The listing builds one solid part. Answer for the finished solid, in the listing's coordinates (mm). A direction names the side the tool comes from. Give positions to 0.01 mm unless a question says otherwise; leave off trailing zeros. Write each loop counter-clockwise with the first axis right and the second up, starting at its lowest first coordinate (ties: lowest second). Pieces come first, ordered by that corner, then holes. Notation, with made-up numbers: (27, 49) -> (69, 49) arc R17 cw to (69, 56) -> close; hole circle Ø6 at (3, 24.25). An arc over 180 degrees is marked (long way). Put each result on its own line as item: value. Start each with the question number.
1) Find the intervals of material crossed by line 1 along X through (y, z) = (2, -3.5); line 2 along X through (y, z) = (2.3, 14); line 3 along X through (y, z) = (2.6, 5), in increasing order. Write a range as from..to.
2) A cutting plane is placed at C-C (y = 0.8). Give the number of separate pieces and of enclosed holes in the cut face, then the cut area to 3 significant figures.
3) A cutting plane is placed at B-B (x = 7). Write down the section's boundary in (y, z) (3 decimals), then the cut area to 3 significant figures.
4) For a pull along Z with two mould halves and no side action, classify faces 1 (the flat face through (29.366, 1.565, 6.476)), 2 (the flat face through (20.58, 1.57, -4.71)), 3 (the flat face through (28.63, 1.57, 8.7)) as released by +Z, released by -Z, zero draft, split by the parting line, or undercut.
5) A cutting plane is placed at D-D (z = 7.75). Write down the section's boundary in (x, y) (3 decimals), then the cut area to 3 significant figures.
6) Flat-ended cylindrical pins translate along their axes: pin 1 Ø2 at (x, z) = (5.5, 3) entering from -Y; pin 2 Ø1.6 at (x, y) = (-3.5, 1) entering from -Z. Find the tip coordinate at first contact, or state that the pin passes through.
7) A cutting plane is placed at A-A (x = 0.72). Write down the section's boundary in (y, z) (1 decimal).
8) For faces 4 (the cylindrical face through (26.784, 1.565, 8.433)), 5 (the flat face through (24.23, 1.57, -3.77)), 6 (the flat face through (15.044, 1.565, 12.893)), 7 (the flat face through (29.262, 1.565, 2.712)), determine the directions among +Z, -Z, +X, -X, +Y, -Y from which every point of the face is accessible in a straight line to the end or side of a thin tool.
from build123d import *

# Parameters (mm, degrees)
CROQUIS1_R              = 1.5875
SALIENTE_EXTRUIR1_DEPTH = 3.175
SALIENTE_EXTRUIR2_START = -3.175
CROQUIS2_R              = 7.5
CROQUIS2_R_2            = 1.5875
SALIENTE_EXTRUIR2_DEPTH = 3.175
SALIENTE_EXTRUIR3_START = -3.175
SALIENTE_EXTRUIR3_DEPTH = 3.175
CORTAR_EXTRUIR4_START   = -10
CORTAR_EXTRUIR4_DEPTH   = 10
MATRIZC1_COUNT          = 8
MATRIZC1_ANGLE          = 259
REDONDEO1_R             = 1
ESQUISSE1_R             = 1.59
ENL_V_MAT_EXTRU_1_DEPTH = 36.494905734


with BuildPart() as part:
    # Croquis1 → Saliente-Extruir1 (new body)
    with BuildSketch(Plane(origin=(0, 0, 0), x_dir=(1, 0, 0), z_dir=(0, 1, 0))):
        with BuildLine():
            Line((-20, 0), (20, 0))
            ThreePointArc((20, 0), (24.7625, -4.7625), (20, -9.525))
            Line((20, -9.525), (-20, -9.525))
            ThreePointArc((-20, -9.525), (-24.7625, -4.7625), (-20, 0))
        make_face()
        with Locations(Location((-20, -4.7625, 0), (0, 0, 270))):
            Circle(CROQUIS1_R, mode=Mode.SUBTRACT)
        with Locations(Location((20, -4.7625, 0), (0, 0, 270))):
            Circle(CROQUIS1_R, mode=Mode.SUBTRACT)
    extrude(amount=SALIENTE_EXTRUIR1_DEPTH)

    # Croquis2 → Saliente-Extruir2 (add)
    with BuildSketch(Plane(origin=(0, 3.175, 0), x_dir=(1, 0, 0), z_dir=(0, 1, 0)).offset(SALIENTE_EXTRUIR2_START)):
        with Locations((20, -4.7625)):
            Circle(CROQUIS2_R)
        with Locations(Location((20, -4.7625, 0), (0, 0, 270))):
            Circle(CROQUIS2_R_2, mode=Mode.SUBTRACT)
    extrude(amount=SALIENTE_EXTRUIR2_DEPTH)

    # Croquis8 → Saliente-Extruir3 (add)
    with BuildSketch(Plane(origin=(0, 3.175, 0), x_dir=(1, 0, 0), z_dir=(0, 1, 0)).offset(SALIENTE_EXTRUIR3_START)):
        with BuildLine():
            Line((11.607813982, 3.461471902), (14.206158981, 0))
            ThreePointArc((14.206158981, 0), (15.121179891, 0.933736858), (16.184441281, 1.694396442))
            Line((16.184441281, 1.694396442), (13.163387879, 4.793819098))
            ThreePointArc((13.163387879, 4.793819098), (12.356515163, 4.161604411), (11.607813982, 3.461471902))
        make_face()
    saliente_extruir3 = extrude(amount=SALIENTE_EXTRUIR3_DEPTH)

    # Croquis9 → Cortar-Extruir4 (cut)
    with BuildSketch(Plane(origin=(0, 3.175, 0), x_dir=(1, 0, 0), z_dir=(0, 1, 0)).offset(CORTAR_EXTRUIR4_START)):
        with BuildLine():
            ThreePointArc((12.35651523, 4.161604469), (11.974526132, 3.819706546), (11.607813982, 3.461471902))
            Line((11.607813982, 3.461471902), (12.19397403, 2.680599255))
            ThreePointArc((12.19397403, 2.680599255), (11.982381708, 3.453243741), (12.35651523, 4.161604469))
        make_face()
        with BuildLine():
            ThreePointArc((13.163387879, 4.793819098), (12.753054069, 4.486514795), (12.35651523, 4.161604469))
            ThreePointArc((12.35651523, 4.161604469), (13.113956627, 4.422436237), (13.844906618, 4.094621057))
            Line((13.844906618, 4.094621057), (13.163387879, 4.793819098))
        make_face()
    cortar_extruir4 = extrude(amount=CORTAR_EXTRUIR4_DEPTH, mode=Mode.SUBTRACT)

    # MatrizC1: Saliente-Extruir3, Cortar-Extruir4 ×8 about axis
    matrizc1_axis = Axis((20, 0, 4.7625), (0, -1, 0))
    add([saliente_extruir3.rotate(matrizc1_axis, i * MATRIZC1_ANGLE / (MATRIZC1_COUNT - 1)) for i in range(1, MATRIZC1_COUNT)])
    add([cortar_extruir4.rotate(matrizc1_axis, i * MATRIZC1_ANGLE / (MATRIZC1_COUNT - 1)) for i in range(1, MATRIZC1_COUNT)], mode=Mode.SUBTRACT)

    # Redondeo1
    # the kernel refuses this fillet: 1 mm, written as the material it adds along each edge
    with BuildSketch(Plane(origin=(27.395406089, 0, 3.514313802), x_dir=(0.12009264391370789, 0, 0.9927626891044079), z_dir=(0, 1, 0)), Plane(origin=(26.657411119, 0, 8.216320666), x_dir=(-0.501549250802915, 0, 0.8651290938461349), z_dir=(0, 1, 0)), Plane(origin=(23.238283761, 0, 11.527373856), x_dir=(-0.9212027273713431, 0, 0.389082941136718), z_dir=(0, 1, 0)), Plane(origin=(18.515005687, 0, 12.114016299), x_dir=(-0.9698611692594302, 0, -0.243658187555294), z_dir=(0, 1, 0)), Plane(origin=(14.389777858, 0, 9.739990082), x_dir=(-0.6279284118017822, 0, -0.7782711029275668), z_dir=(0, 1, 0)), Plane(origin=(16.184441281, 0, -1.694396442), x_dir=(0.8837864601497757, 0, -0.4678904710035554), z_dir=(0, 1, 0)), Plane(origin=(20.838616598, 0, -2.690467342), x_dir=(0.9874067650142349, 0, 0.15820202402031353), z_dir=(0, 1, 0)), Plane(origin=(25.155056708, 0, -0.685012307), x_dir=(0.6933697506528057, 0, 0.7205819792915072), z_dir=(0, 1, 0))) as redondeo1_piece_1:
        with BuildLine():
            CenterArc((0.748840141, 0.998904162), REDONDEO1_R, 196.368950511, 70.948483307)
            Line((-0.210626698, 0.717082614), (0, 0))
            ThreePointArc((0, 0), (0.351018816, 0.008218784), (0.702037632, 0))
        make_face()
    extrude(amount=3.175)
    with BuildSketch(Plane(origin=(26.522503707, 0, 1.06021079), x_dir=(0.9617717559465732, 0, -0.2738523132336944), z_dir=(0, 1, 0)), Plane(origin=(27.437196341, 0, 5.731061088), x_dir=(0.9329135130884484, 0, 0.36010050971495355), z_dir=(0, 1, 0)), Plane(origin=(25.35671448, 0, 10.011843767), x_dir=(0.5283439627642348, 0, 0.8490304217226758), z_dir=(0, 1, 0)), Plane(origin=(21.11892846, 0, 12.178563585), x_dir=(-0.0890050127232042, 0, 0.9960311780813601), z_dir=(0, 1, 0)), Plane(origin=(16.430517523, 0, 11.358619681), x_dir=(-0.6705090902301596, 0, 0.7419013141373477), z_dir=(0, 1, 0)), Plane(origin=(18.238976871, 0, -2.527822183), x_dir=(0.0018564846529317855, 0, -0.9999982767308818), z_dir=(0, 1, 0)), Plane(origin=(22.981009808, 0, -2.119620351), x_dir=(0.6032966406304949, 0, -0.7975168734289948), z_dir=(0, 1, 0))) as redondeo1_piece_2:
        with BuildLine():
            CenterArc((0.747376131, 1), REDONDEO1_R, 199.051516693, 70.948483307)
            ThreePointArc((-0.197849332, 0.673581828), (-0.091039016, 0.339107144), (0, 0))
            Line((0, 0), (0.747376131, 0))
        make_face()
    extrude(amount=3.175)
    with BuildSketch(Plane(origin=(14.206158981, 3.175, 0), x_dir=(-1, 0, 0), z_dir=(0, -1, 0))) as redondeo1_piece_3:
        with BuildLine():
            CenterArc((REDONDEO1_R * 2.00103600097, REDONDEO1_R), REDONDEO1_R, 143.106368796, 126.893631204)
            Line((REDONDEO1_R * 1.20128460683, REDONDEO1_R * 1.6003313315), (0, 0))
            Line((0, 0), (REDONDEO1_R * 2.00103600097, 0))
        make_face()
    extrude(amount=3.175)
    with BuildSketch(Plane(origin=(14.206158981, 3.175, 9.525), x_dir=(-1, 0, 0), z_dir=(0, -1, 0))) as redondeo1_piece_4:
        with BuildLine():
            CenterArc((0.454646298, -1), REDONDEO1_R, 90, 47.317031956)
            ThreePointArc((-0.280469857, -0.322058824), (-0.137942125, -0.163026135), (0, 0))
            Line((0, 0), (0.454646298, 0))
        make_face()
    extrude(amount=3.175)

    # Esquisse1 → Enlèv. mat.-Extru.1 (cut, through all)
    with BuildSketch(Plane(origin=(0, 3.175, 0), x_dir=(1, 0, 0), z_dir=(0, 1, 0))):
        with Locations(Location((0.72, -4.7625, 0), (0, 0, 270))):
            Circle(ESQUISSE1_R)
        with Locations(Location((-4.02, -4.7625, 0), (0, 0, 270))):
            Circle(ESQUISSE1_R)
    extrude(amount=-ENL_V_MAT_EXTRU_1_DEPTH, mode=Mode.SUBTRACT)


solid = part.part
Reply:
1. line 1: x = 11.99..14.42, 18.24..20.74, 24.03..26.76
1. line 2: x = 12.74..14.01, 18.59..20.96, 25.26..27.13
1. line 3: x = -24.76..-21.57, -18.43..-5.59, -2.45..-0.85, 2.29..18.43, 21.57..27.5
2. separate pieces: 1
2. enclosed holes: 4
2. area: 574 mm2
3. outline: (0, 0) -> (3.175, 0) -> (3.175, 9.525) -> (0, 9.525) -> close
3. area: 30.2 mm2
4. face 1: undercut
4. face 2: released by -Z
4. face 3: released by +Z
5. outline: (-23.709, 0) -> (31.242, 0) -> (31.242, 3.175) -> (-23.709, 3.175) -> close
5. area: 174 mm2
6. pin 1: stops at y = 0
6. pin 2: stops at z = 0
7. outline: (0, 0) -> (3.2, 0) -> (3.2, 3.2) -> (0, 3.2) -> close; (0, 6.4) -> (3.2, 6.4) -> (3.2, 9.5) -> (0, 9.5) -> close
8. face 4: +Y, -Y
8. face 5: -Z, +Y, -Y
8. face 6: +Z, +Y, -Y
8. face 7: +X, +Y, -Y
